The listing builds one solid part. Answer for the finished solid, in the listing's coordinates (mm). A direction names the side the tool comes from. Round coordinates to 2 decimals unless told otherwise and drop trailing zeros. Loops run counter-clockwise (first coordinate to the right, second up) from the corner with the lowest first, then second, coordinate; pieces in that order, holes last. Notation, with made-up numbers: (17, 57) -> (22, 57) arc R15 ccw to (22, 74) -> close; hole circle Ø11 at (-27.5, -32.75). An arc over 180 degrees is marked (long way). One line per question, with ' | ' between items.
from build123d import *

# Parameters (mm, degrees)
F1_DEPTH      = 3.175
F3_DEPTH      = 3.175
F4_W          = 3.175
F4_H          = 3.175
F5_DEPTH      = 50.8
F5_DEPTH_BACK = 50.8


# Not quite as in the source:
# - an extrude ends at something that could not be found from the text; its depth is read off the source's solid


with BuildPart() as f1:
    # F0 (on Top) → F1 (new body)
    with BuildSketch(Plane.XY):
        with BuildLine():
            Line((-50.8, 0), (50.8, 0))
            ThreePointArc((50.8, 0), (0, 50.8), (-50.8, 0))
        make_face()
    extrude(amount=F1_DEPTH)

    # F2 (on face) → F3 (join)
    with BuildSketch(Plane.XZ):
        with BuildLine():
            ThreePointArc((50.8, 3.175), (0, 53.975), (-50.8, 3.175))
            Line((-50.8, 3.175), (50.8, 3.175))
        make_face()
    extrude(amount=F3_DEPTH)

    # F4 (on Right) → F5 (join, two sides)
    with BuildSketch(Plane.YZ) as f5_sk:
        with Locations((-1.5875, 1.5875)):
            Rectangle(F4_W, F4_H)
    extrude(amount=F5_DEPTH)
    extrude(f5_sk.sketch, amount=-F5_DEPTH_BACK)


solid = f1.part
Q1. A cutting plane is placed at D-D on z = 27. Give the vertices of the cut face in (x, y) (3 decimals).
Numbers:
outline: (-44.867, -3.175) -> (44.867, -3.175) -> (44.867, 0) -> (-44.867, 0) -> close
Q2. Find the intervals of material crossed by line 1 (Y direction, x = 24.5, z = 11.5) (3 decimals); line 2 (Z direction, x = -14, y = 9) (3 decimals), in increasing order. Write a range as from..to.
Numbers:
line 1: -3.175..0 | line 2: 0..3.175
Q3. A cutting plane is placed at B-B on z = 4.5. Give the vertices of the cut face in (x, y) (3 decimals).
Numbers:
outline: (-50.783, -3.175) -> (50.783, -3.175) -> (50.783, 0) -> (-50.783, 0) -> close
Q4. A cutting plane is placed at A-A on x = 0. Give the vertices of the cut face in (y, z) (3 decimals).
Numbers:
outline: (-3.175, 0) -> (50.8, 0) -> (50.8, 3.175) -> (0, 3.175) -> (0, 53.975) -> (-3.175, 53.975) -> close
Q5. For faces 1 (the face through (-1, 0, 23)), 2 (the face through (-50.8, -2, 2)), determine the directions among +Z, -Z, +X, -X, +Y, -Y from which every point of the face is accessible in a straight line to the end or side of a thin tool.
Numbers:
face 1: +Z, +X, -X, +Y | face 2: +Z, -Z, -X, +Y, -Y
Q6. A cutting plane is placed at C-C on x = 20. Give the vertices of the cut face in (y, z) (3 decimals).
Numbers:
outline: (-3.175, 0) -> (46.697, 0) -> (46.697, 3.175) -> (0, 3.175) -> (0, 49.872) -> (-3.175, 49.872) -> close
Q7. Given pin 1 Ø1.5 at (x, z) = (-5.5, 36.5) entering from +Y; pin 2 Ø8 at (x, y) = (26.5, 39.5) entering from +Z (3 decimals), each flat-ended and moving along its own axis, determine where each tip first touches the part or whether it passes through.
Numbers:
pin 1: y = 0 | pin 2: z = 3.175
